Read the model definition and answer for the solid it produces. Units are mm, in the model's axes. A direction names the side the tool comes from. Coordinates: 2 decimals unless noted, no trailing zeros. Write each loop counter-clockwise with the first axis right and the second up, starting at its lowest first coordinate (ties: lowest second). Pieces come first, ordered by that corner, then holes. Notation, with made-up numbers: M 68,1 L 89,1 A30 ccw 89,32 Z; hole C 46,22 d6. An arc over 180 degrees is marked long. Use a Markdown table: item, result. Add a question column.
Autodesk Inventor part; units mm, degrees
ref_plane "РабПлоскость1" through (0, 11, 0) normal (0, 1, 0) x (-1, 0, 0)
ref_plane "YZ Plane" through (0, 0, 0) normal (1, 0, 0) x (0, 1, 0)
ref_plane "XY Plane" through (0, 0, 0) normal (0, 0, 1) x (1, 0, 0)
sketch "Эскиз1" plane through (0, 0, 0) normal (0, 0, 1) x (1, 0, 0)
  line L0 (0, 0) -> (0, 7.5)
  line L1 (22.4142, 6.5) -> (25.4, 6.5)
  line L2 (27, 8.1) -> (27, 15)
  line L3 (27, 15) -> (67, 15)
  line L4 (100, 10) -> (100, 0)
  line L5 (100, 0) -> (0, 0)
  line L6 (0, 7.5) -> (21, 7.5)
  line L7 (21, 7.5) -> (21.7071, 6.7929)
  line L8 (100, 10) -> (67, 10)
  line L9 (67, 15) -> (67, 10)
  arc A0 (21.7071, 6.7929) -> (22.4142, 6.5) centre (22.4142, 7.5) ccw
  arc A1 (25.4, 6.5) -> (27, 8.1) centre (25.4, 8.1) ccw
  point P0 (22, 6.5)
  point P1 (27, 6.5)
  point P2 (67, 12.5)
  dimension "d0" = 27
  dimension "d4" = 100
  dimension "d14" = 6.5
  dimension "d21" = 135
  dimension "d22" = 1
  dimension "d23" = 5
  dimension "d26" = 10
  dimension "d27" = 40
  dimension "d28" = 15
  dimension "d70" = 1
  dimension "d71" = 1.6
revolve "Вращение1" add sketch "Эскиз1" angle 360 about axis through (100, 0, 0) along (-1, 0, 0)
sketch "Эскиз2" plane through (0, 0, 0) normal (0, 0, 1) x (1, 0, 0)
  point P0 (0, 0)
sketch "Эскиз4" plane through (0, 0, 0) normal (0, 0, 1) x (1, 0, 0)
  circle A0 centre (90, 0) radius 2.5
  line L0 (100, -10) -> (100, 10)
  point P0 (0, 0)
  dimension "d38" = 10
  dimension "d39" = 5
  dimension "d40" = 90
extrude "Выдавливание2" cut sketch "Эскиз4" along normal through all both and the other way through all
thread "Резьба1"
chamfer "Фаска1" distance 2 angle 45 1 edges at (0, -7.5, 0)
chamfer "Фаска2" distance 2.5 angle 45 1 edges at (67, -15, 0) measured on face at (67, 13.0912, 1.9943)
chamfer "Фаска3" distance 2 angle 45 1 edges at (100, -10, 0) measured on face at (100, -0.4018, -2.9244)
chamfer "Фаска4" distance 2.5 angle 45 1 edges at (27, -15, 0) measured on face at (27, 12.5547, 1.1966)
ref_plane "РабПлоскость1" through (0, 11, 0) normal (0, 1, 0) x (-1, 0, 0)
sketch "Эскиз5" plane through (0, 11, 0) normal (0, 1, 0) x (-1, 0, 0)
  line L0 (-29.5, -15) -> (-29.5, 15)
  line L1 (11.4, 0) -> (-68.4, 0)
  line L2 (-27, -8.5) -> (-27, 8.5)
  arc A0 (-41, -4) -> (-41, 4) centre (-41, 0) ccw
  line L3 (-41, -4) -> (-53, -4)
  arc A1 (-53, 4) -> (-53, -4) centre (-53, 0) ccw
  line L4 (-41, 4) -> (-53, 4)
  point P0 (0, 0)
  dimension "d66" = 10
  dimension "d67" = 20
  dimension "d68" = 8
  dimension "d69" = 4
extrude "Выдавливание3" cut sketch "Эскиз5" along normal blind 4
properties part number "Вал"
Item 1: Find section C-C on x = 36. Give the vertices of the cut face in (y, z).
Item 2: For faces 4 (the cylindrical face through (23.928, -5.158, -3.955)), 5 (the flat face through (27, 3, 8)), 6 (the flat face through (67, -0.1, -10.2)), 7 (the cylindrical face through (37, 13, 0)), 8 (the cylindrical face through (87.5, 0.1, 0.1)), determine the directions among +Z, -Z, +X, -X, +Y, -Y from which every point of the face is accessible in a straight line to the end or side of a thin tool.
Item 3: Each of these flat-tipped pins is pushed along its axis until it touches: pin 1 (5 mm diameter, centred on x = 68.5, y = 11.5, fed in from +Z); pin 2 (1.5 mm diameter, centred on x = 25, y = 8.5, fed in from -Z); pin 3 (5 mm diameter, centred on x = 32.5, z = 3.5, fed in from -Y); pin 4 (8 mm diameter, centred on y = 7, z = -10, fed in from -X). Where does it stop, or does it pass through?
Item 4: Consider probe 1 along X at (y, z) = (0, -2); probe 2 along Y at (x, z) = (90, -2); probe 3 along X at (y, z) = (10, 6). Determine where each line is inside the solid, lowest interval first.
Item 5: Find section D-D on x = 90. Give the vertices of the cut face in (y, z).
Item 6: Determine the mould class of faces 1 (the conical face through (99.87, -1.06, -8.06)), 2 (the cylindrical face through (57, 13, 0)), 3 (the flat face through (0, 0, 0)) for opening direction X: pulls with the +X half, pulls with the -X half, needs draft (parallel to the pull), parting line crosses it, or undercut.
Geometry says:
| question | item | result |
|---|---|---|
| 1 | outline | C 0,0 d30 |
| 2 | face 4 | none |
| 2 | face 5 | -X |
| 2 | face 6 | +X |
| 2 | face 7 | +Y |
| 2 | face 8 | +Z, -Z |
| 3 | pin 1 | stops at z = 8.31 |
| 3 | pin 2 | passes through |
| 3 | pin 3 | stops at y = -14.97 |
| 3 | pin 4 | stops at x = 27 |
| 4 | probe 1 | x = 0 to 87.5, 92.5 to 100 |
| 4 | probe 2 | y = -9.8 to -2.5, 2.5 to 9.8 |
| 4 | probe 3 | x = 27 to 67 |
| 5 | outline | M -2.5,-9.68 L -2.5,9.68 A10 ccw Z; M 2.5,-9.68 A10 ccw 2.5,9.68 Z |
| 6 | face 1 | pulls with the +X half |
| 6 | face 2 | undercut |
| 6 | face 3 | pulls with the -X half |
